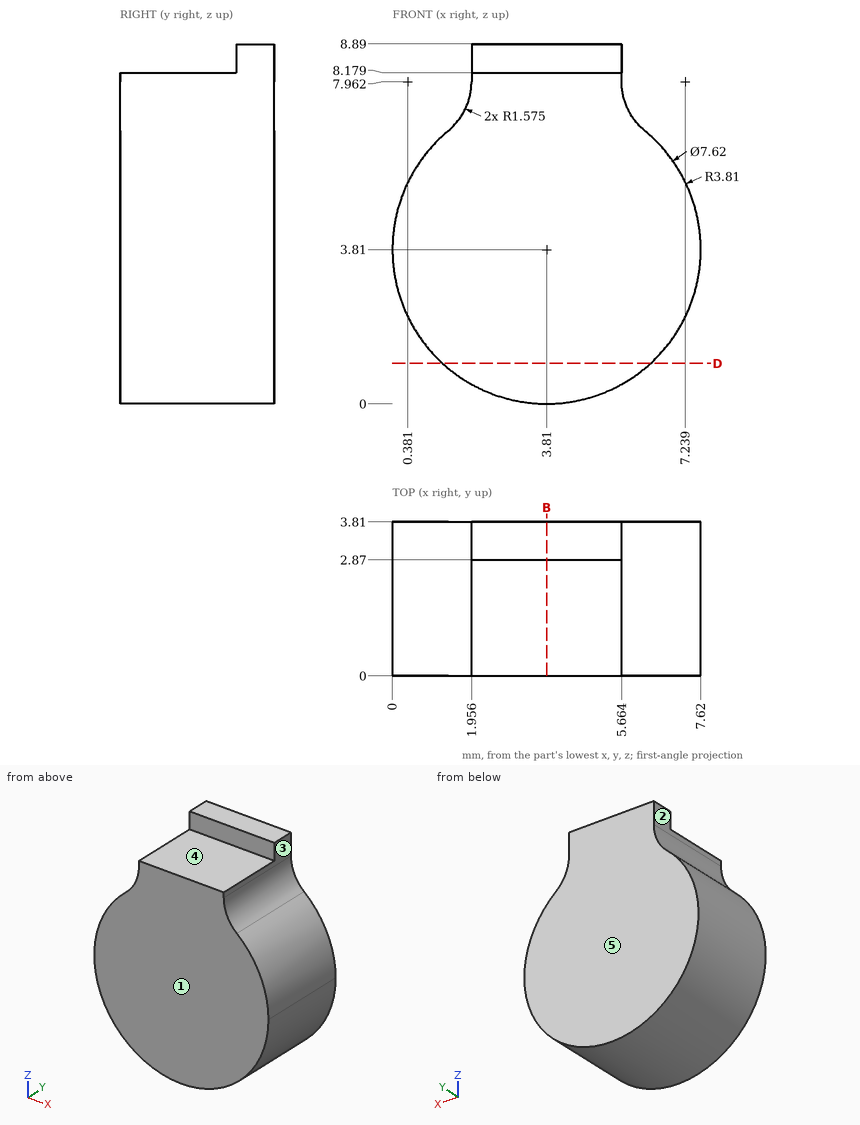
Job drawing, mm, ordinate dimensions from the low corner. One solid piece. A direction names the side the tool comes from. Give positions to 0.01 mm unless a question says otherwise; leave off trailing zeros. Order: outer loops, then holes, each group sorted by start corner. A loop starts at its lowest first (then second) coordinate and runs counter-clockwise, first axis right, second up. Notation, with made-up numbers: M 62,-27.5 L 121,-27.5 A15 ccw 121,-17.5 Z; hole C -13.75,37.5 d2. An arc over 180 degrees is marked long. Return JSON: item names as keys, results as strings.
Q1. Wall check: probe 1 along X at (y, z) = (1.25, 8); probe 2 along Y at (x, z) = (4, 8.25); probe 3 along X at (y, z) = (0.8, 7). Give the ranges that are in metal, low to high. Write a range as from..to.
Answer list:
{"probe 1": "x = 1.96..5.66", "probe 2": "y = 2.87..3.81", "probe 3": "x = 1.63..5.99"}
Q2. Flat gauge pins, fed straight in: pin 1 (0.9 mm diameter, centred on x = 3, y = 1.5, fed in from +Z); pin 2 (1 mm diameter, centred on x = 5, y = 3, fed in from -Z); pin 3 (1 mm diameter, centred on y = 1.5, z = 8.5, fed in from -X). Where does each tip first touch, or does it go through?
Answer list:
{"pin 1": "stops at z = 8.18", "pin 2": "stops at z = 0.06", "pin 3": "stops at x = 1.96"}
Q3. 3-axis set-ups, long thin cutter, end or side, ignore diameter. For the marked faces 1, 2, 3, 4 and 5: which of +Z, -Z, +X, -X, +Y, -Y reach the whole face in a straight line?
Answer list:
{"face 1": "+Z, -Z, +X, -X, -Y", "face 2": "+Z, -X, +Y, -Y", "face 3": "+Z, +X, +Y, -Y", "face 4": "+Z, +X, -X, -Y", "face 5": "+Z, -Z, +X, -X, +Y"}
Q4. Band-saw the part on B-B (x = 3.81). Give the cut face in (y, z).
Answer list:
{"outline": "M 0,0 L 3.81,0 L 3.81,8.89 L 2.87,8.89 L 2.87,8.18 L 0,8.18 Z"}
Q5. Band-saw the part on D-D (z = 1). Give the cut face in (x, y).
Answer list:
{"outline": "M 1.24,0 L 6.38,0 L 6.38,3.81 L 1.24,3.81 Z"}
